Here's how the part is built. I have some questions about the finished solid (model axes, mm). Coordinates: 2 decimals unless noted, no trailing zeros. Write each loop counter-clockwise with the first axis right and the second up, starting at its lowest first coordinate (ties: lowest second). Pieces come first, ordered by that corner, then holes. Notation, with made-up numbers: (56, -39.5) -> (99, -39.5) arc R25 ccw to (99, -12.5) -> close; hole circle Ø7 at (82, -27.75). An arc over 180 degrees is marked (long way). Put each result on its own line as item: value.
```python
from build123d import *

# Parameters (mm, degrees)
SKETCH1_W           = 60
SKETCH1_H           = 60
SKETCH1_R           = 2.5
BOSS_EXTRUDE2_DEPTH = 5
SKETCH4_W           = 30
SKETCH4_H           = 60.044205022
SKETCH4_R           = 2.5
SKETCH4_H_2         = 60
BOSS_EXTRUDE5_DEPTH = 5
FILLET1_R           = 30


with BuildPart() as part:
    # Sketch1 → Boss-Extrude2 (new body)
    with BuildSketch(Plane(origin=(0, 0, 0), x_dir=(1, 0, 0), z_dir=(0, 1, 0))):
        with Locations((30, 30)):
            Rectangle(SKETCH1_W, SKETCH1_H)
        with Locations(Location((30, 40.020671676, 0), (0, 0, 270))):
            Circle(SKETCH1_R, mode=Mode.SUBTRACT)
        with Locations(Location((20, 30.020671676, 0), (0, 0, 270))):
            Circle(SKETCH1_R, mode=Mode.SUBTRACT)
        with Locations(Location((30, 20.020671676, 0), (0, 0, 270))):
            Circle(SKETCH1_R, mode=Mode.SUBTRACT)
        with Locations(Location((40, 30.020671676, 0), (0, 0, 270))):
            Circle(SKETCH1_R, mode=Mode.SUBTRACT)
        with Locations(Location((30, 30.020671676, 0), (0, 0, 270))):
            Circle(SKETCH1_R, mode=Mode.SUBTRACT)
    extrude(amount=BOSS_EXTRUDE2_DEPTH)

    # Sketch4 → Boss-Extrude5 (add)
    # profile 1 of 2: a face of its own
    with BuildSketch(Plane(origin=(0, 0, 0), x_dir=(1, 0, 0), z_dir=(0, 1, 0))):
        with Locations((75, 29.977897489)):
            Rectangle(SKETCH4_W, SKETCH4_H)
        with Locations(Location((63, 29.977897489, 0), (0, 0, 270))):
            Circle(SKETCH4_R, mode=Mode.SUBTRACT)
        with Locations(Location((75, 29.977897489, 0), (0, 0, 270))):
            Circle(SKETCH4_R, mode=Mode.SUBTRACT)
    # profile 2 of 2: a face of its own
    with BuildSketch(Plane(origin=(0, 0, 0), x_dir=(1, 0, 0), z_dir=(0, 1, 0))):
        with Locations((-15, 30)):
            Rectangle(SKETCH4_W, SKETCH4_H_2)
        with Locations(Location((-3, 29.977897489, 0), (0, 0, 270))):
            Circle(SKETCH4_R, mode=Mode.SUBTRACT)
        with Locations(Location((-15, 29.977897489, 0), (0, 0, 270))):
            Circle(SKETCH4_R, mode=Mode.SUBTRACT)
    extrude(amount=BOSS_EXTRUDE5_DEPTH)

    # Fillet1
    fillet1_edges = [part.edges().sort_by_distance(p)[0] for p in [
        (-30, 2.5, 0),
        (-30, 2.5, -60),
        (90, 2.5, 0.044205022),
        (90, 2.5, -60),
    ]]
    fillet(fillet1_edges, radius=FILLET1_R - 0.0001)  # a hair under: the kernel refuses the full size


solid = part.part
```
Item 1: If we mould it in two halves opening along Z, with no side actions, what happens to faces 1 (the cylindrical face through (32.11, 2.46, -18.68)), 2 (the cylindrical face through (-20.979, 2.535, -51.445)), 3 (the flat face through (29, 0, -24))? For each: released by +Z, released by -Z, zero draft, split by the parting line, or undercut.
Output:
face 1: undercut
face 2: released by -Z
face 3: zero draft
Item 2: For P1, Ø8, axis at x = -15, z = -29.98, coming from the -Y side; P2, Ø4.5, axis at x = 20, z = -30.02, coming from the -Y side, each with a flat end and sliding along its axis, tell me the tip position at first contact or that it passes through.
Output:
P1: stops at y = 0
P2: passes through
Item 3: Imagine slicing it at A-A on y = 1.45. State how many separate pieces and enclosed holes the cut face has, then the cut area to 3 significant figures.
Output:
separate pieces: 1
enclosed holes: 9
area: 6,250 mm²
Item 4: Imagine slicing it at C-C on x = 63. Write out the boundary of the cut face in (y, z).
Output:
outline: (0, -59.85) -> (5, -59.85) -> (5, -32.48) -> (0, -32.48) -> close; (0, -27.48) -> (5, -27.48) -> (5, -0.11) -> (0, -0.11) -> close
Item 5: Imagine slicing it at B-B on x = 20. Write out the boundary of the cut face in (y, z), then the cut area to 3 significant figures.
Output:
outline: (0, -60) -> (5, -60) -> (5, -32.52) -> (0, -32.52) -> close; (0, -27.52) -> (5, -27.52) -> (5, 0) -> (0, 0) -> close
area: 275 mm²
Item 6: Imagine slicing it at D-D on z = -10. Write out the boundary of the cut face in (x, y).
Output:
outline: (-22.36, 0) -> (82.4, 0) -> (82.4, 5) -> (-22.36, 5) -> close
Item 7: Please list where these lines run through material, in increasing order: line 1 along X through (y, z) = (1.65, -39); line 2 along Z through (x, y) = (29, 0.95); line 3 along Z through (x, y) = (53.5, 0.95). Write a range as from..to.
Output:
line 1: x = -28.62..27.72, 32.28..88.62
line 2: z = -60..-42.31, -37.73..-32.31, -27.73..-22.31, -17.73..0
line 3: z = -60..0
